Input: part model. Units: mm. Frame: model coordinates. A direction names the side the tool comes from. Round coordinates to 2 decimals unless told otherwise and drop trailing zeros. Write each loop counter-clockwise with the first axis right and the second up, starting at its lowest first coordinate (ties: lowest second). Pieces come first, ordered by that corner, then holes. Notation, with made-up numbers: M 16.25,-23.75 L 66.25,-23.75 A27 ccw 66.25,3.25 Z; hole C -2,49.25 d7. An arc over 180 degrees is marked long. Write each question's results on one line, items separated by ' | '. Start each with the question number.
```python
from build123d import *

# Parameters (mm, degrees)
SKETCH4_R           = 12.5
BOSS_EXTRUDE3_DEPTH = 22
SKETCH5_R           = 5
CUT_EXTRUDE1_DEPTH  = 37
SKETCH6_R           = 5
BOSS_EXTRUDE4_DEPTH = 102
SKETCH7_R           = 2.5
BOSS_EXTRUDE5_DEPTH = 4
SKETCH8_R           = 4
BOSS_EXTRUDE6_DEPTH = 8


with BuildPart() as part:
    # Sketch4 → Boss-Extrude3 (new body)
    with BuildSketch(Plane.XY):
        with Locations((0, 1.214400682)):
            Circle(SKETCH4_R)
    extrude(amount=BOSS_EXTRUDE3_DEPTH)

    # Sketch5 → Cut-Extrude1 (cut)
    with BuildSketch(Plane(origin=(13, 0, 0), x_dir=(0, 0, -1), z_dir=(1, 0, 0))):
        with Locations((-11.919301613, 1.755166336)):
            Circle(SKETCH5_R)
    extrude(amount=-CUT_EXTRUDE1_DEPTH, mode=Mode.SUBTRACT)

    # Sketch6 → Boss-Extrude4 (add)
    with BuildSketch(Plane.XY.offset(22)):
        with Locations((0, 1.805272807)):
            Circle(SKETCH6_R)
    extrude(amount=BOSS_EXTRUDE4_DEPTH)

    # Sketch7 → Boss-Extrude5 (add)
    with BuildSketch(Plane.XY.offset(124)):
        with Locations((0, 1.74135251)):
            Circle(SKETCH7_R)
    extrude(amount=BOSS_EXTRUDE5_DEPTH)

    # Sketch8 → Boss-Extrude6 (add)
    with BuildSketch(Plane.XY.offset(128)):
        with Locations((0, 1.74135251)):
            Circle(SKETCH8_R)
    extrude(amount=BOSS_EXTRUDE6_DEPTH)


solid = part.part
```
1. Contact query for flat-ended pins moving along their axis: P1, Ø3, axis at x = -3, z = 109.5, coming from the +Y side; P2, Ø10, axis at x = -9, y = 8, coming from the +Z side; P3, Ø10, axis at x = 3.5, z = 89.5, coming from the -Y side; P4, Ø9, axis at y = 1.76, z = 11.92, coming from the -X side. Output: stop coordinate, or through.
2. Draft query along Y for faces 4 (the face through (0.17, -2.68, 9.61)), 5 (the face through (0, -4, 22)), 6 (the face through (2.69, 6.02, 72.29)). Return one class per face: +Y half, -Y half, draft (parallel to the pull), parting line (faces both ways), or undercut.
3. Cut plane D-D on y = 10.25. Output: boundary loops of the cut face in (x, z), and give its area (3 significant figures).
4. Cut plane A-A on x = 0. Output: boundary loops of the cut face in (y, z).
5. Line query: L1, parallel to Z at x = 3, y = -8.75; L2, parallel to Z at x = 1.5, y = -2.25; L3, parallel to Z at x = -11, y = 5.5. Output: solid intervals per line, ascending. Write a range as from..to.
6. Access query for faces 1 (the face through (2, 0, 124)), 2 (the face through (5.768, -9.875, 10.846)), 3 (the face through (3.695, 0.209, 131.944)). Directions: +Z, -Z, +X, -X, +Y, -Y. A direction counts if a zero-diameter tool reaches every point of the face in a straight line with its end or side. Return the directions, or none.
7. Cut plane C-C on x = 9.25. Output: boundary loops of the cut face in (y, z).
8. Cut plane B-B on z = 62. Output: boundary loops of the cut face in (x, y), and give its area (3 significant figures).
Answers follow:
1) P1: stops at y = 6.57 | P2: stops at z = 22 | P3: stops at y = -3.19 | P4: passes through
2) face 4: undercut | face 5: draft | face 6: parting line
3) outline: M -8.64,0 L 8.64,0 L 8.64,22 L -8.64,22 Z | area: 380 mm2
4) outline: M -11.29,0 L 13.71,0 L 13.71,22 L 6.81,22 L 6.81,124 L 4.24,124 L 4.24,128 L 5.74,128 L 5.74,136 L -2.26,136 L -2.26,128 L -0.76,128 L -0.76,124 L -3.19,124 L -3.19,22 L -11.29,22 Z; hole C 1.76,11.92 d10
5) L1: z = 0..22 | L2: z = 0..8.93, 14.91..124 | L3: z = 0..8.61, 15.23..22
6) face 1: none | face 2: +Z, -Z | face 3: +Z
7) outline: M -7.19,0 L 9.62,0 L 9.62,22 L -7.19,22 Z; hole C 1.76,11.92 d10
8) outline: C 0,1.81 d10 | area: 78.5 mm2
